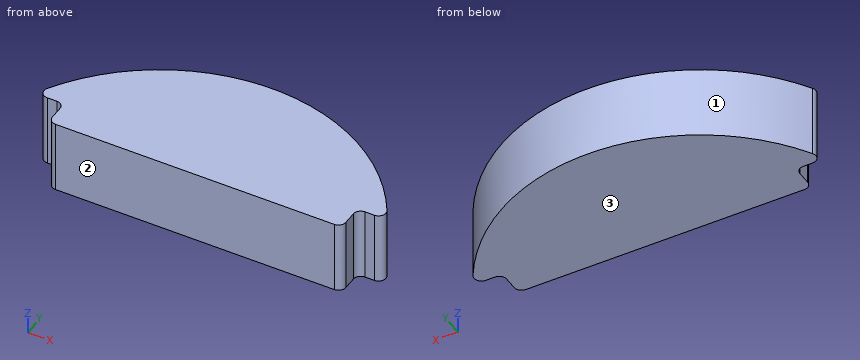
from build123d import *

# Parameters (mm, degrees)
BOSS_EXTRU_1_DEPTH = 50
COQUE1_T           = 2


with BuildPart() as part:
    # Esquisse1 → Boss.-Extru.1 (new body)
    with BuildSketch(Plane.XY):
        with BuildLine():
            Line((-79.110112943, 0), (110.889887057, 0))
            ThreePointArc((110.889887057, 0), (114.425420963, 1.464466094), (115.889887057, 5))
            Line((115.889887057, 5), (115.889887057, 14.2))
            ThreePointArc((115.889887057, 14.2), (117.354353151, 17.735533906), (120.889887057, 19.2))
            Line((120.889887057, 19.2), (127.386676949, 19.2))
            ThreePointArc((127.386676949, 19.2), (131.737258082, 21.735767095), (131.675015022, 26.771022476))
            ThreePointArc((131.675015022, 26.771022476), (15.889887057, 92.353415616), (-99.895240907, 26.771022476))
            ThreePointArc((-99.895240907, 26.771022476), (-99.957483967, 21.735767095), (-95.606902834, 19.2))
            Line((-95.606902834, 19.2), (-89.110112943, 19.2))
            ThreePointArc((-89.110112943, 19.2), (-85.574579037, 17.735533906), (-84.110112943, 14.2))
            Line((-84.110112943, 14.2), (-84.110112943, 5))
            ThreePointArc((-84.110112943, 5), (-82.645646849, 1.464466094), (-79.110112943, 0))
        make_face()
    extrude(amount=BOSS_EXTRU_1_DEPTH)

    # Coque1 (no face opened: a closed hollow body)
    add(offset(amount=-COQUE1_T, mode=Mode.PRIVATE), mode=Mode.SUBTRACT)


solid = part.part
Verification items for the finished model (mm, model axes). Face numbers are marked on the shaded views. Round coordinates to 2 decimals unless told otherwise and drop trailing zeros. Write each loop counter-clockwise with the first axis right and the second up, starting at its lowest first coordinate (ties: lowest second). Pieces come first, ordered by that corner, then holes.
(1) Section check A-A (z = 16). Enter the section's corners in (x, y).
Returned:
outline: (-99.9, 26.77) arc R5 ccw to (-95.61, 19.2) - (-89.11, 19.2) arc R5 cw to (-84.11, 14.2) - (-84.11, 5) arc R5 ccw to (-79.11, 0) - (110.89, 0) arc R5 ccw to (115.89, 5) - (115.89, 14.2) arc R5 cw to (120.89, 19.2) - (127.39, 19.2) arc R5 ccw to (131.68, 26.77) arc R135 ccw to start; hole (-98.18, 25.74) arc R3 ccw to (-95.61, 21.2) - (-89.11, 21.2) arc R7 cw to (-82.11, 14.2) - (-82.11, 5) arc R3 ccw to (-79.11, 2) - (110.89, 2) arc R3 ccw to (113.89, 5) - (113.89, 14.2) arc R7 cw to (120.89, 21.2) - (127.39, 21.2) arc R3 ccw to (129.96, 25.74) arc R133 ccw to start
(2) Section check B-B (x = -60). Enter the section's corners in (y, z), plus the area to 3 significant figures.
Returned:
outline: (0, 0) - (69, 0) - (69, 50) - (0, 50) - close; hole (2, 2) - (66.58, 2) - (66.58, 48) - (2, 48) - close
area: 480 mm2
(3) Material ranges on line 1 (Z direction, x = 93, y = 61.5); line 2 (X direction, y = 14, z = 39.5); line 3 (X direction, y = 31, z = 40.5), recorded low to high.
Returned:
line 1: z = 0 to 2, 48 to 50
line 2: x = -84.11 to -82.11, 113.89 to 115.89
line 3: x = -97.25 to -94.86, 126.64 to 129.03
(4) Section check C-C (y = 33.5). Enter the section's corners in (x, z).
Returned:
outline: (-95.59, 0) - (127.36, 0) - (127.36, 50) - (-95.59, 50) - close; hole (-93.15, 2) - (124.93, 2) - (124.93, 48) - (-93.15, 48) - close
(5) Depth check by flat-ended pin: pin 1 Ø1.9 at (x, z) = (123, 13.5) entering from -Y; pin 2 Ø5 at (x, z) = (123.5, 31) entering from +Y; pin 3 Ø1.9 at (x, z) = (-91, 25.5) entering from +Y. Enter the tip coordinate at first touch or a pass-through.
Returned:
pin 1: stops at y = 19.2
pin 2: stops at y = 42.07
pin 3: stops at y = 41.03
(6) Mould release check, pull along Y, two halves, no side actions. Record for the marked faces 1, 2 and 3: pulls with the +Y half, pulls with the -Y half, needs draft (parallel to the pull), parting line crosses it, or undercut.
Returned:
face 1: pulls with the +Y half
face 2: pulls with the -Y half
face 3: needs draft
